from build123d import *

# Parameters (mm, degrees)
CROQUIS1_W              = 45
CROQUIS1_H              = 20
SALIENTE_EXTRUIR1_DEPTH = 25
VACIADO5_T              = 1
REDONDEO1_R             = 1
CORTAR_EXTRUIR1_START   = -10
CORTAR_EXTRUIR1_DEPTH   = 5
CHAFL_N2_SIZE           = 1


with BuildPart() as part:
    # Croquis1 → Saliente-Extruir1 (new body)
    with BuildSketch(Plane(origin=(0, 0, 0), x_dir=(1, 0, 0), z_dir=(0, 1, 0))):
        Rectangle(CROQUIS1_W, CROQUIS1_H)
    extrude(amount=SALIENTE_EXTRUIR1_DEPTH)

    # Vaciado5
    vaciado5_openings = [part.faces().sort_by_distance(p)[0] for p in [
        (0, 25, 0),
    ]]
    offset(amount=VACIADO5_T, openings=vaciado5_openings, kind=Kind.INTERSECTION)

    # Redondeo1
    # the kernel refuses this fillet: 1 mm, written as the material it takes off along each edge
    with BuildSketch(Plane(origin=(-23.5, -3.5, -11), x_dir=(1, 0, 0), z_dir=(0, 1, 0)), Plane(origin=(23.5, -3.5, -11), x_dir=(0, 0, 1), z_dir=(0, 1, 0))) as redondeo1_piece_1:
        with BuildLine():
            CenterArc((REDONDEO1_R, -REDONDEO1_R), REDONDEO1_R, 90, 90)
            Line((0, -REDONDEO1_R), (0, 0))
            Line((0, 0), (REDONDEO1_R, 0))
        make_face()
    extrude(amount=31, mode=Mode.SUBTRACT)

    # Croquis2 → Cortar-Extruir1 (cut)
    with BuildSketch(Plane.XY.offset(CORTAR_EXTRUIR1_START)):
        with BuildLine():
            ThreePointArc((17.768716436, 19.753391932), (15.925504733, 17.743649431), (13.30186607, 17))
            Line((13.30186607, 17), (-13.30186607, 17))
            ThreePointArc((-13.30186607, 17), (-15.925504733, 17.743649431), (-17.768716436, 19.753391932))
            Line((-17.768716436, 19.753391932), (-18.332567601, 20.87447701))
            ThreePointArc((-18.332567601, 20.87447701), (-19.090471642, 21.981034188), (-20.115254744, 22.846312707))
            Line((-20.115254744, 22.846312707), (-23.5, 25))
            Line((-23.5, 25), (23.5, 25))
            Line((23.5, 25), (20.115254744, 22.846312707))
            ThreePointArc((20.115254744, 22.846312707), (19.090471642, 21.981034188), (18.332567601, 20.87447701))
            Line((18.332567601, 20.87447701), (17.768716436, 19.753391932))
        make_face()
    extrude(amount=-CORTAR_EXTRUIR1_DEPTH, mode=Mode.SUBTRACT)

    # Chaflán1
    # the kernel refuses this chamfer: 1 mm, written as the material it takes off along each edge
    with BuildSketch(Plane(origin=(-22.5, 25, -10), x_dir=(0.027495876610585647, -0.9996219169112968, 0), z_dir=(0, 0, 1))) as chafl_n1_piece_1:
        with BuildLine():
            Line((1.028673195, 0), (-0.056547155, -1.027117794))
            Line((-0.056547155, -1.027117794), (-0.076539593, -1.026567876))
            ThreePointArc((-0.076539593, -1.026567876), (-0.034129227, -0.51339783), (-0.019992438, 0.000549918))
            Line((-0.019992438, 0.000549918), (0.000549918, 0.019992438))
            ThreePointArc((0.000549918, 0.019992438), (0.514497665, 0.00585565), (1.029223113, 0.019992438))
            Line((1.029223113, 0.019992438), (1.028673195, 0))
        make_face()
    extrude(amount=20, mode=Mode.SUBTRACT)

    # Chaflán2
    # the kernel refuses this chamfer: 1 mm, written as the material it takes off along each edge
    with BuildSketch(Plane(origin=(22.5, 25, 10), x_dir=(-0.027495876610585647, -0.9996219169112968, 0), z_dir=(0, 0, -1))) as chafl_n2_piece_1:
        Polygon((CHAFL_N2_SIZE * 0.999621916911, -CHAFL_N2_SIZE * 0.0274958766106), (-CHAFL_N2_SIZE * 0.0274958766106, -CHAFL_N2_SIZE * 0.999621916911), (0, 0), align=None)
    extrude(amount=20, mode=Mode.SUBTRACT)


solid = part.part
The model under review builds one solid part; all positions refer to its coordinate system, in mm. A direction names the side the tool comes from. Give positions to 0.01 mm unless a question says otherwise; leave off trailing zeros. Order: outer loops, then holes, each group sorted by start corner. A loop starts at its lowest first (then second) coordinate and runs counter-clockwise, first axis right, second up. Notation, with made-up numbers: M 88.25,9.25 L 92.25,9.25 A25 cw 92.25,25.25 Z; hole C 62.25,-3.5 d3. An arc over 180 degrees is marked long. One line per question, with ' | ' between items. Start each with the question number.
1) Consider section D-D, the plane y = 20.25. Give the boundary of the cut face in (x, z).
2) Consider section A-A, the plane y = 3.25. Give the boundary of the cut face in (x, z).
3) Consider section C-C, the plane z = -3.5. Give the boundary of the cut face in (x, y).
4) Clearance check with a flat-ended pin moving along its axis: P1, Ø0.5, axis at x = -2.5, z = -10.5, coming from the +Y side. State where the tip first meets the part, or that it passes through.
5) Wall thickness on L1, parallel to Z at x = 2, y = 14.25; L2, parallel to X at y = 16.5, z = -7.75; L3, parallel to Y at x = -10, z = 8.25: over which ranges is each line inside the solid? List them lowest first. Write a range as from..to.
6) For faces 1 (the face through (-23.199, 11.818, -10.715)), 2 (the face through (-18.05, 20.31, -10.49)), 3 (the face through (-23, 24.5, -0.1)), list the 3-axis set-ups (+Z, -Z, +X, -X, +Y, -Y) from which the entire face can be reached by the end or side of a thin tool; tool diameter is ignored.
7) Consider section B-B, the plane x = 2. Give the boundary of the cut face in (y, z).
Found:
1) outline: M -23.5,-10 A1 ccw -22.5,-11 L -18.02,-11 L -18.02,-10 L -22.5,-10 L -22.5,10 L 22.5,10 L 22.5,-10 L 18.02,-10 L 18.02,-11 L 22.5,-11 A1 ccw 23.5,-10 L 23.5,11 L -23.5,11 Z
2) outline: M -23.5,-10 A1 ccw -22.5,-11 L 22.5,-11 A1 ccw 23.5,-10 L 23.5,11 L -23.5,11 Z; hole M -22.5,-10 L 22.5,-10 L 22.5,10 L -22.5,10 Z
3) outline: M -23.5,-1 L 23.5,-1 L 23.5,25 L 22.5,24 L 22.5,0 L -22.5,0 L -22.5,24 L -23.5,25 Z
4) P1: stops at y = 17
5) L1: z = -11..-10, 10..11 | L2: x = -23.5..-22.5, 22.5..23.5 | L3: y = -1..0
6) face 1: -Z, -X, +Y, -Y | face 2: -Z, +Y | face 3: +Y
7) outline: M -1,-11 L 17,-11 L 17,-10 L 0,-10 L 0,10 L 25,10 L 25,11 L -1,11 Z
